CAD build for the part. Positions are in the model's coordinates, mm. A direction names the side the tool comes from. Give positions to 0.01 mm unless a question says otherwise; leave off trailing zeros. Loops run counter-clockwise (first coordinate to the right, second up) from the corner with the lowest first, then second, coordinate; pieces in that order, holes last.
```python
from build123d import *

# Parameters (mm, degrees)
SKETCH2_R         = 1.4986
CENTER_HOLE_DEPTH = 16.24


with BuildPart() as part:
    # Sketch1 → Revolve1 (revolve)
    with BuildSketch(Plane(origin=(0, 0, 0), x_dir=(1, 0, 0), z_dir=(0, 1, 0))):
        Polygon((0, 0), (0, 4.699), (1.524, 4.699), (1.524, 2.38125), (7.874, 2.38125), (7.874, 3.14325), (15.24, 3.14325), (15.24, 0), align=None)
    revolve(axis=Axis((15.24, 0, 0), (-1, 0, 0)))

    # Sketch2 → Center-Hole (cut, through all)
    with BuildSketch(Plane.ZY):
        Circle(SKETCH2_R)
    extrude(amount=-CENTER_HOLE_DEPTH, mode=Mode.SUBTRACT)

    # Sketch3 → Cut-Revolve1 (revolve, cut)
    with BuildSketch(Plane(origin=(0, 0, 0), x_dir=(1, 0, 0), z_dir=(0, 1, 0))):
        with BuildLine():
            Line((1.524, 4.699), (0, 4.699))
            Line((0, 4.699), (0, 1.4986))
            ThreePointArc((0, 1.4986), (0.548299529, 3.200562129), (1.524, 4.699))
        make_face()
    revolve(axis=Axis((0, 0, 0), (1, 0, 0)), mode=Mode.SUBTRACT)


solid = part.part
```
1. Tool access for faces 1 (the face through (7.51, 0.45, 1.43)), 2 (the face through (4.74, 1.45, 1.89)): list every direction of +Z, -Z, +X, -X, +Y, -Y with a clear straight run to the whole face (end or side of a thin tool).
Responses:
face 1: +X, -X
face 2: none
2. Saw through at B-B, the plane x = 14. List the corners of the cut face in (y, z), and give its area (3 significant figures).
Responses:
outline: circle Ø6.29 at (0, 0); hole circle Ø3 at (0, 0)
area: 24.0 mm2
3. Drop flat-ended pins along their axis: pin 1 (3 mm diameter, centred on y = 1, z = -0.5, fed in from -X); pin 2 (4 mm diameter, centred on x = 6.5, z = 0.5, fed in from +Y). Give the stop position or say it passes through.
Responses:
pin 1: stops at x = 0
pin 2: stops at y = 3.14
4. Pull direction X, two halves, no side cores. Call faces 3 (the face through (1.524, 2, -2)), 4 (the face through (11.61, 3.07, 0.68)): released by +X, released by -X, zero draft, split by the parting line, or undercut.
Responses:
face 3: undercut
face 4: zero draft
5. Saw through at A-A, the plane x = 2.5. List the corners of the cut face in (y, z), and give its area (3 significant figures).
Responses:
outline: circle Ø4.76 at (0, 0); hole circle Ø3 at (0, 0)
area: 10.8 mm2
6. Probe line 1 along Y through (x, z) = (6.75, 0); line 2 along Z through (x, y) = (9, 0). List the from-to ranges inside material, lowest first.
Responses:
line 1: y = -2.38 to -1.5, 1.5 to 2.38
line 2: z = -3.14 to -1.5, 1.5 to 3.14
